from build123d import *

# Parameters (mm, degrees)
SKETCH_1_R      = 19
SKETCH_1_R_2    = 17
EXTRUDE_1_DEPTH = 148


with BuildPart() as part:
    # 草图1 → 凸台-拉伸1 (new body)
    with BuildSketch(Plane(origin=(0, 0, 0), x_dir=(1, 0, 0), z_dir=(0, 1, 0))):
        with Locations(Location((0, 0, 0), (0, 0, 270))):
            Circle(SKETCH_1_R)
        with Locations(Location((0, 0, 0), (0, 0, 270))):
            Circle(SKETCH_1_R_2, mode=Mode.SUBTRACT)
    extrude(amount=EXTRUDE_1_DEPTH)

    # 草图6 → 旋转1 (revolve)
    with BuildSketch(Plane.XY, mode=Mode.PRIVATE) as revolve_1_sk:
        Polygon((-19, 0), (-17, 0), (-4.027808676, -4.632925473), (-1.5, -38), (-2.5, -38), (-5, -5), align=None)
    revolve(revolve_1_sk.sketch.rotate(Axis((0, 0, 0), (0, -1, 0)), 270), axis=Axis((0, 0, 0), (0, -1, 0)))


solid = part.part
Geometry: final body of the model. Coordinates: model frame, mm. A direction names the side the tool comes from. Give positions to 0.01 mm unless a question says otherwise; leave off trailing zeros. Write each loop counter-clockwise with the first axis right and the second up, starting at its lowest first coordinate (ties: lowest second). Pieces come first, ordered by that corner, then holes. Notation, with made-up numbers: (-27, 8) -> (-18, 8) arc R26 ccw to (-18, 38) -> close; hole circle Ø7 at (48, -21). An arc over 180 degrees is marked (long way). Answer as a JSON object with one key per item and string values.
1. Mould query, pull axis X, two halves, no side actions, for faces 3 (the conical face through (1.44, -21.27, 3.48)), 4 (the flat face through (2, -38, 0)), 5 (the conical face through (-1.4, -4.41, 4.44)). Classes: pulls with the +X half, pulls with the -X half, needs draft (parallel to the pull), parting line crosses it, or undercut.
Ans:
{"face 3": "parting line crosses it", "face 4": "needs draft", "face 5": "undercut"}
2. Ray query, probe 1 along X at (y, z) = (88, 0); probe 2 along Z at (x, y) = (3, 63); probe 3 along Z at (x, y) = (-10.5, 61). Return the intervals inside material, ascending. Write a range as from..to.
Ans:
{"probe 1": "x = -19..-17, 17..19", "probe 2": "z = -18.76..-16.73, 16.73..18.76", "probe 3": "z = -15.84..-13.37, 13.37..15.84"}
3. Cut plane C-C on y = -18. Output: boundary loops of the cut face in (x, z), and give its area (3 significant figures).
Ans:
{"outline": "circle Ø8.03 at (0, 0); hole circle Ø6.03 at (0, 0)", "area": "22.1 mm^2"}
4. Cut plane A-A on x = 0. Output: boundary loops of the cut face in (y, z).
Ans:
{"outline": "(-38, -2.5) -> (-5, -5) -> (0, -19) -> (148, -19) -> (148, -17) -> (0, -17) -> (-4.63, -4.03) -> (-38, -1.5) -> close; (-38, 1.5) -> (-4.63, 4.03) -> (0, 17) -> (148, 17) -> (148, 19) -> (0, 19) -> (-5, 5) -> (-38, 2.5) -> close"}
5. Contact query for flat-ended pins moving along their axis: pin 1 (3 mm diameter, centred on x = -4.5, z = 5.5, fed in from -Y); pin 2 (12 mm diameter, centred on y = 80, z = -9, fed in from -X); pin 3 (2 mm diameter, centred on x = 13.5, y = -5, fed in from +Z); pin 4 (1.5 mm diameter, centred on x = 6.5, y = 39, fed in from +Z). Output: stop coordinate, or through.
Ans:
{"pin 1": "stops at y = -4.78", "pin 2": "stops at x = -18.76", "pin 3": "passes through", "pin 4": "stops at z = 18.11"}
6. Cut plane B-B on y = 48. Output: boundary loops of the cut face in (x, z), and give its area (3 significant figures).
Ans:
{"outline": "circle Ø38 at (0, 0); hole circle Ø34 at (0, 0)", "area": "226 mm^2"}
7. Access query for faces 1 (the cylindrical face through (16.855, 72.964, -2.213)), 2 (the conical face through (3.575, -4.687, -4.663)). Directions: +Z, -Z, +X, -X, +Y, -Y. A direction counts if a zero-diameter tool reaches every point of the face in a straight line with its end or side. Return the directions, or none.
Ans:
{"face 1": "+Y", "face 2": "-Y"}
